```python
from build123d import *

# Parameters (mm, degrees)
BOSS_EXTRUDE1_DEPTH = 8
SKETCH2_R           = 5
BOSS_EXTRUDE2_DEPTH = 29
FILLET1_R           = 2
SKETCH3_R           = 1.55
CUT_EXTRUDE1_DEPTH  = 15.6
FILLET2_R           = 1
SKETCH5_R           = 2.0875
CUT_EXTRUDE3_DEPTH  = 3
CUT_EXTRUDE4_REACH  = 10
SKETCH6_R           = 1.25
SKETCH7_R           = 0.5
CUT_EXTRUDE5_DEPTH  = 0.5


with BuildPart() as part:
    # Sketch1 → Boss-Extrude1 (new body)
    with BuildSketch(Plane(origin=(0, 0, 0), x_dir=(1, 0, 0), z_dir=(0, 1, 0))):
        Polygon((7.3, -4.214656965), (7.3, 4.214656965), (0, 8.42931393), (-7.3, 4.214656965), (-7.3, -4.214656965), (0, -8.42931393), align=None)
    extrude(amount=BOSS_EXTRUDE1_DEPTH)

    # Sketch2 → Boss-Extrude2 (add)
    with BuildSketch(Plane.XZ):
        Circle(SKETCH2_R)
        with BuildLine():
            Line((-1.5, 1.451776928), (-1.5, -1.451776928))
            ThreePointArc((-1.5, -1.451776928), (2.0875, 0), (-1.5, 1.451776928))
        make_face(mode=Mode.SUBTRACT)
    extrude(amount=BOSS_EXTRUDE2_DEPTH)

    # Fillet1
    fillet1_edges = [part.edges().sort_by_distance(p)[0] for p in [
        (-5, 0, 0),
    ]]
    fillet(fillet1_edges, radius=FILLET1_R)

    # Sketch3 → Cut-Extrude1 (cut, through all)
    with BuildSketch(Plane(origin=(7.3, 0, 0), x_dir=(0, 0, -1), z_dir=(1, 0, 0))):
        with Locations((-0.085343035, 3.85)):
            Circle(SKETCH3_R)
    extrude(amount=-CUT_EXTRUDE1_DEPTH, mode=Mode.SUBTRACT)

    # Fillet2
    fillet2_edges = [part.edges().sort_by_distance(p)[0] for p in [
        (0, 4, 8.42931393),
        (-7.3, 4, 4.214656965),
        (-7.3, 4, -4.214656965),
        (0, 4, -8.42931393),
        (7.3, 4, -4.214656965),
        (7.3, 4, 4.214656965),
        (3.65, 8, -6.321985448),
        (-3.65, 8, -6.321985448),
        (-7.3, 8, 0),
        (-3.65, 8, 6.321985448),
        (3.65, 8, 6.321985448),
        (7.3, 8, 0),
    ]]
    fillet(fillet2_edges, radius=FILLET2_R)

    # Sketch5 → Cut-Extrude3 (cut)
    with BuildSketch(Plane.XZ.offset(29)):
        Circle(SKETCH5_R)
    extrude(amount=-CUT_EXTRUDE3_DEPTH, mode=Mode.SUBTRACT)

    # Sketch6 → Cut-Extrude4 (cut, up to next)
    with BuildSketch(Plane.XZ, mode=Mode.PRIVATE) as cut_extrude4_sk1:
        Circle(SKETCH6_R)
    cut_extrude4_tool1 = extrude(cut_extrude4_sk1.sketch, amount=-CUT_EXTRUDE4_REACH, mode=Mode.PRIVATE) & part.part
    add(cut_extrude4_tool1.solids().sort_by_distance((0, 0, 0))[0], mode=Mode.SUBTRACT)

    # Sketch7 → Cut-Extrude5 (cut)
    with BuildSketch(Plane(origin=(3.65, 0, -6.321985448), x_dir=(-0.866025404, 0, -0.5), z_dir=(0.5, 0, -0.866025404))):
        with Locations((0, 3.5)):
            Circle(SKETCH7_R)
    extrude(amount=-CUT_EXTRUDE5_DEPTH, mode=Mode.SUBTRACT)


solid = part.part
```
Build history of the part. All positions in model axes, mm. A direction names the side the tool comes from. Coordinates: 2 decimals unless noted, no trailing zeros. Order: outer loops, then holes, each group sorted by start corner. A loop starts at its lowest first (then second) coordinate and runs counter-clockwise, first axis right, second up. Notation, with made-up numbers: (22.5, 30) -> (47.5, 30) arc R15 cw to (47.5, 36) -> close; hole circle Ø3 at (-14.75, -19). An arc over 180 degrees is marked (long way). Answer in a Markdown table with one row per item. Add a question column.
Q1. Which spindle directions (+Z, -Z, +X, -X, +Y, -Y) get a long thin tool onto all of the face, cutting with end or side? Do faces 1 (the face through (-3.69, 3.45, 6.3)), 2 (the face through (-6, 0, 4)). Say none if no direction does.
Q2. Drop flat-ended pins along their axis: pin 1 (1 mm diameter, centred on x = -1.5, y = -6, fed in from +Z); pin 2 (0.9 mm diameter, centred on y = -16, z = -0.5, fed in from +X); pin 3 (1.8 mm diameter, centred on x = 0.5, z = 0.5, fed in from -Y). Give the stop position or say it passes through.
Q3. Band-saw the part on C-C, the plane y = -1. List the corners of the cut face in (x, z) (1 decimal).
Q4. Mould opens along Z. For faces 3 (the face through (-1.5, -13, 0)), 4 (the face through (7.17, 3.55, 4.13)), 5 (the face through (-7.3, 2, 0)) say: +Z half, -Z half, draft (parallel to the pull), parting line (faces both ways), or undercut.
Q5. Wall check: line 1 along X through (y, z) = (1, 0); line 2 along Z through (x, y) = (0, -21); line 3 along Z through (x, y) = (0, 1.7). Give the ranges that are in metal, low to high. Write a range as [from, to].
Q6. Band-saw the part on A-A, the plane y = -14. List the corners of the cut face in (x, z) (1 decimal).
Q7. Band-saw the part on B-B, the plane z = 0. List the corners of the cut face in (x, y).
Answers follow:
| question | item | result |
|---|---|---|
| 1 | face 1 | +Z, -X, +Y, -Y |
| 1 | face 2 | -Y |
| 2 | pin 1 | z = 4.9 |
| 2 | pin 2 | x = 5 |
| 2 | pin 3 | y = 0 |
| 3 | outline | circle Ø10.5 at (0, 0); hole (-1.5, -1.5) arc R2.1 ccw (long way) to (-1.5, 1.5) -> close |
| 4 | face 3 | undercut |
| 4 | face 4 | +Z half |
| 4 | face 5 | draft |
| 5 | line 1 | [-7.3, -1.25], [1.25, 7.3] |
| 5 | line 2 | [-5, -2.09], [2.09, 5] |
| 5 | line 3 | [-8.27, -1.25], [1.25, 8.27] |
| 6 | outline | circle Ø10 at (0, 0); hole (-1.5, -1.5) arc R2.1 ccw (long way) to (-1.5, 1.5) -> close |
| 7 | outline | (-7.3, 0) -> (-7, 0) arc R2 cw to (-5, -2) -> (-5, -29) -> (-2.09, -29) -> (-2.09, -26) -> (-1.5, -26) -> (-1.5, 0) -> (-1.25, 0) -> (-1.25, 2.3) -> (-7.3, 2.3) -> close; (-7.3, 5.4) -> (7.3, 5.4) -> (7.3, 7) arc R1 ccw to (6.3, 8) -> (-6.3, 8) arc R1 ccw to (-7.3, 7) -> close; (1.25, 0) -> (2.09, 0) -> (2.09, -29) -> (5, -29) -> (5, -2) arc R2 cw to (7, 0) -> (7.3, 0) -> (7.3, 2.3) -> (1.25, 2.3) -> close |
